Check sheet for the drawn part. Datum: minimum x, y, z corner. Units: mm. A direction names the side the tool comes from. Give positions to 0.01 mm unless a question says otherwise; leave off trailing zeros. Loops run counter-clockwise (first coordinate to the right, second up) from the corner with the lowest first, then second, coordinate; pieces in that order, holes last. Notation, with made-up numbers: (74, 26.5) - (116, 26.5) arc R30 cw to (116, 52.5) - close; hole circle Ø7 at (38, -39). An arc over 180 degrees is marked (long way). One line per item, written item: value. Start each with the question number.
1. Gauge pin test, flat ends, axial feed: pin 1 (1.5 mm diameter, centred on x = 16, z = 29, fed in from -Y); pin 2 (1 mm diameter, centred on y = 10.5, z = 32, fed in from -X). Record the tip position at first contact, or that the pin passes through.
2. Sectioned sample at A-A (z = 8.75). Record the cut outline in (x, y), plus the area to 3 significant figures.
3. Mould release check, pull along X, two halves, no side actions. Record for the marked faces 1, 2, 3 and 4: pulls with the +X half, pulls with the -X half, needs draft (parallel to the pull), parting line crosses it, or undercut.
4. Scan lines: L1, parallel to X at y = 19.5, z = 13; L2, parallel to Y at x = 31.5, z = 16; L3, parallel to X at y = 14.5, z = 7. Record each from-to range of solid material in increasing order. Write a range as [from, to].
5. Sectioned sample at D-D (z = 32.25). Record the cut outline in (x, y).
6. Sectioned sample at C-C (y = 8). Record the cut outline in (x, z).
7. Sectioned sample at B-B (y = 14.5). Record the cut outline in (x, z), plus the area to 3 significant figures.
8. Access from +Z, -Z, +X, -X, +Y, -Y to the whole of each face (thin tool, end or side, straight path). Record for the marked faces 5 and 6.
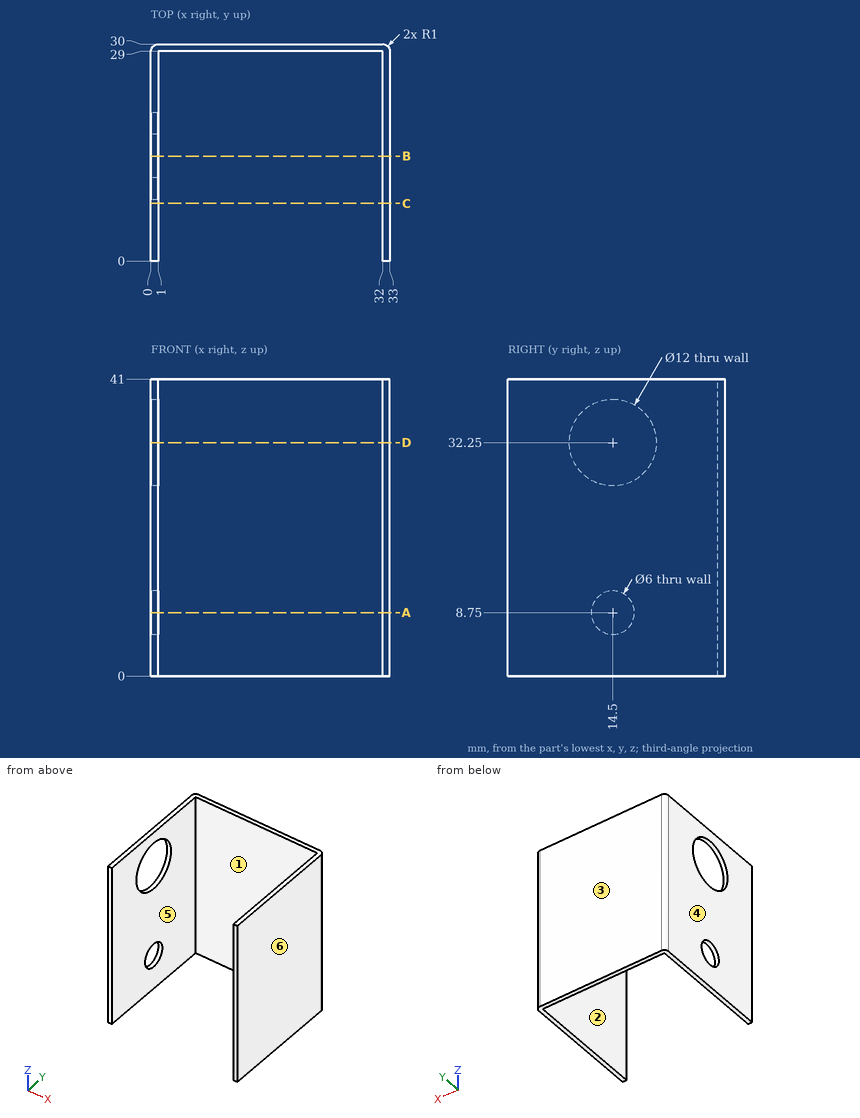
Results are:
1. pin 1: stops at y = 29
1. pin 2: stops at x = 32
2. outline: (0, 0) - (1, 0) - (1, 11.5) - (0, 11.5) - close; (0, 17.5) - (1, 17.5) - (1, 29) - (32, 29) - (32, 0) - (33, 0) - (33, 29) arc R1 ccw to (32, 30) - (1, 30) arc R1 ccw to (0, 29) - close
2. area: 84.6 mm^2
3. face 1: undercut
3. face 2: undercut
3. face 3: needs draft
3. face 4: pulls with the -X half
4. L1: x = [0, 1], [32, 33]
4. L2: y = [29, 30]
4. L3: x = [32, 33]
5. outline: (0, 0) - (1, 0) - (1, 8.5) - (0, 8.5) - close; (0, 20.5) - (1, 20.5) - (1, 29) - (32, 29) - (32, 0) - (33, 0) - (33, 29) arc R1 ccw to (32, 30) - (1, 30) arc R1 ccw to (0, 29) - close
6. outline: (0, 0) - (1, 0) - (1, 41) - (0, 41) - close; (32, 0) - (33, 0) - (33, 41) - (32, 41) - close
7. outline: (0, 0) - (1, 0) - (1, 5.75) - (0, 5.75) - close; (0, 11.75) - (1, 11.75) - (1, 26.25) - (0, 26.25) - close; (0, 38.25) - (1, 38.25) - (1, 41) - (0, 41) - close; (32, 0) - (33, 0) - (33, 41) - (32, 41) - close
7. area: 64.0 mm^2
8. face 5: +Z, -Z, -Y
8. face 6: +Z, -Z, +X, +Y, -Y
